The model under review builds one solid part; all positions refer to its coordinate system, in mm. Face numbers are marked on the shaded views. A direction names the side the tool comes from. Give positions to 0.01 mm unless a question says otherwise; leave off trailing zeros. Loops run counter-clockwise (first coordinate to the right, second up) from the corner with the lowest first, then second, coordinate; pieces in that order, holes last. Notation, with made-up numbers: M 70.5,61 L 105.5,61 A32 cw 105.5,88 Z; hole C 30.25,62 d3. An arc over 180 degrees is marked long. Return JSON: item names as keys, results as strings.
```python
from build123d import *

# Parameters (mm, degrees)
SKETCH_3_W          = 50
SKETCH_3_H          = 7
EXTRUDE_1_DEPTH     = 33
EXTRUDE_2_DEPTH     = 33
SKETCH_5_R          = 1.25
CUT_EXTRUDE_1_DEPTH = 8
SKETCH_6_W          = 50
SKETCH_6_H          = 4
CUT_EXTRUDE_2_DEPTH = 40
CUT_EXTRUDE_START   = -8
SKETCH_7_R          = 1.25
CUT_EXTRUDE_3_DEPTH = 8


with BuildPart() as part:
    # 草图3 → 凸台-拉伸1 (new body)
    with BuildSketch(Plane.XY):
        with Locations((25, 25)):
            Rectangle(SKETCH_3_W, SKETCH_3_H)
    extrude(amount=EXTRUDE_1_DEPTH)

    # 草图4 → 凸台-拉伸2 (add)
    with BuildSketch(Plane(origin=(0, 0, 0), x_dir=(-1, 0, 0), z_dir=(0, 0, -1))):
        with BuildLine():
            Line((-50, 21.5), (-50, 11))
            ThreePointArc((-50, 11), (-47.86188219, 17.51667431), (-42.278719262, 21.5))
            Line((-42.278719262, 21.5), (-50, 21.5))
        make_face()
        with BuildLine():
            Line((-7.721280738, 21.5), (0, 21.5))
            Line((0, 21.5), (0, 11))
            ThreePointArc((0, 11), (-2.13811781, 17.51667431), (-7.721280738, 21.5))
        make_face()
        with BuildLine():
            Line((0, 28.5), (0, 39))
            ThreePointArc((0, 39), (-2.13811781, 32.48332569), (-7.721280738, 28.5))
            Line((-7.721280738, 28.5), (0, 28.5))
        make_face()
        with BuildLine():
            Line((-50, 28.5), (-42.278719262, 28.5))
            ThreePointArc((-42.278719262, 28.5), (-47.86188219, 32.48332569), (-50, 39))
            Line((-50, 39), (-50, 28.5))
        make_face()
    extrude(amount=-EXTRUDE_2_DEPTH)

    # 草图5 → 切除-拉伸1 (cut)
    with BuildSketch(Plane(origin=(0, 0, 0), x_dir=(-1, 0, 0), z_dir=(0, 0, -1))):
        with Locations((-46.372516673, 28)):
            Circle(SKETCH_5_R)
        with Locations((-46.372516673, 22)):
            Circle(SKETCH_5_R)
        with Locations((-37.264513071, 25)):
            Circle(SKETCH_5_R)
        with Locations(Location((-3.627483327, 22, 0), (0, 0, 180))):
            Circle(SKETCH_5_R)
        with Locations(Location((-3.627483327, 28, 0), (0, 0, 180))):
            Circle(SKETCH_5_R)
        with Locations(Location((-12.735486929, 25, 0), (0, 0, 180))):
            Circle(SKETCH_5_R)
    extrude(amount=-CUT_EXTRUDE_1_DEPTH, mode=Mode.SUBTRACT)

    # 草图6 → 切除-拉伸2 (cut)
    with BuildSketch(Plane(origin=(0, 0, 0), x_dir=(-1, 0, 0), z_dir=(0, 0, -1))):
        with Locations((-25, 37)):
            Rectangle(SKETCH_6_W, SKETCH_6_H)
        with Locations((-25, 13)):
            Rectangle(SKETCH_6_W, SKETCH_6_H)
    extrude(amount=-CUT_EXTRUDE_2_DEPTH, mode=Mode.SUBTRACT)

    # 草图7 → 切除-拉伸3 (cut)
    with BuildSketch(Plane.XY.offset(33).offset(CUT_EXTRUDE_START)):
        with Locations((3.627483327, 28)):
            Circle(SKETCH_7_R)
        with Locations((3.627483327, 22)):
            Circle(SKETCH_7_R)
        with Locations((12.735486929, 25)):
            Circle(SKETCH_7_R)
        with Locations(Location((46.372516673, 22, 0), (0, 0, 180))):
            Circle(SKETCH_7_R)
        with Locations(Location((46.372516673, 28, 0), (0, 0, 180))):
            Circle(SKETCH_7_R)
        with Locations(Location((37.264513071, 25, 0), (0, 0, 180))):
            Circle(SKETCH_7_R)
    extrude(amount=CUT_EXTRUDE_3_DEPTH, mode=Mode.SUBTRACT)


solid = part.part
```
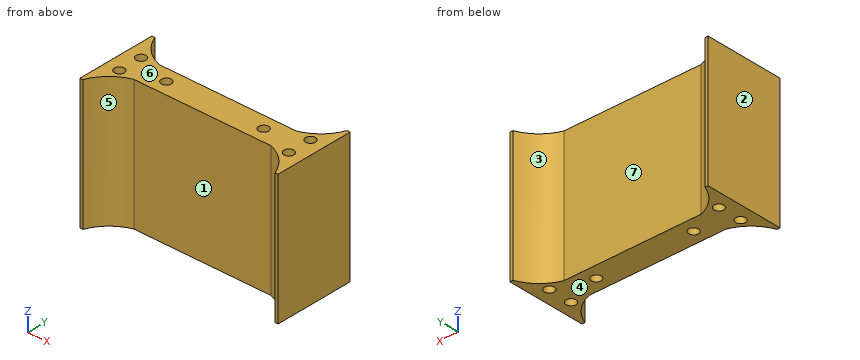
1) Insertion check: pin 1 (2 mm diameter, centred on x = 3.63, y = 28, fed in from +Z); pin 2 (1.2 mm diameter, centred on x = 12.5, y = 25, fed in from -Z); pin 3 (4 mm diameter, centred on x = 31, y = 19, fed in from -Z). Each pin has a flat end and moves straight along its axis. Give the tip position at first contact, or say it passes through.
From the geometry:
{"pin 1": "z = 25", "pin 2": "z = 8", "pin 3": "through"}
2) Consider section B-B on y = 19.5. Write out the cut boundary in (x, z), then the cut area to 3 significant figures.
From the geometry:
{"outline": "M 0,0 L 4.02,0 L 4.02,33 L 0,33 Z; M 45.98,0 L 50,0 L 50,33 L 45.98,33 Z", "area": "265 mm²"}
3) Consider section C-C on y = 25. Write out the cut boundary in (x, z), then the cut area to 3 significant figures.
From the geometry:
{"outline": "M 0,0 L 11.49,0 L 11.49,8 L 13.99,8 L 13.99,0 L 36.01,0 L 36.01,8 L 38.51,8 L 38.51,0 L 50,0 L 50,33 L 38.51,33 L 38.51,25 L 36.01,25 L 36.01,33 L 13.99,33 L 13.99,25 L 11.49,25 L 11.49,33 L 0,33 Z", "area": "1,570 mm²"}
4) Tool access review of the marked faces 5, 6 and 7: name each direction out of +Z, -Z, +X, -X, +Y, -Y from which nothing blocks a thin tool from reaching the whole face with its end or side.
From the geometry:
{"face 5": "+Z, -Z, -Y", "face 6": "+Z, +X, -X, +Y, -Y", "face 7": "+Z, -Z, +Y"}
5) Consider section D-D on z = 23. Write out the cut boundary in (x, y).
From the geometry:
{"outline": "M 0,15 L 0.75,15 A11 cw 7.72,21.5 L 42.28,21.5 A11 cw 49.25,15 L 50,15 L 50,35 L 49.25,35 A11 cw 42.28,28.5 L 7.72,28.5 A11 cw 0.75,35 L 0,35 Z"}
6) The part is to be moulded in two halves that separate along X. For the marked faces 1, 2, 3 and 4, say which applies: released by +X, released by -X, zero draft, split by the parting line, or undercut.
From the geometry:
{"face 1": "undercut", "face 2": "released by -X", "face 3": "undercut", "face 4": "zero draft"}
7) Consider section A-A on z = 27. Write out the cut boundary in (x, y).
From the geometry:
{"outline": "M 0,15 L 0.75,15 A11 cw 7.72,21.5 L 42.28,21.5 A11 cw 49.25,15 L 50,15 L 50,35 L 49.25,35 A11 cw 42.28,28.5 L 7.72,28.5 A11 cw 0.75,35 L 0,35 Z; hole C 3.63,22 d2.5; hole C 3.63,28 d2.5; hole C 12.74,25 d2.5; hole C 37.26,25 d2.5; hole C 46.37,22 d2.5; hole C 46.37,28 d2.5"}
8) Wall thickness on L1, parallel to Y at x = 34, z = 10.5; L2, parallel to X at y = 33.75, z = 11.5; L3, parallel to Y at x = 4.5, z = 29: over which ranges is each line inside the solid? List them lowest first. Write a range as from..to.
From the geometry:
{"L1": "21.5..28.5", "L2": "0..1.33, 48.67..50", "L3": "19.87..21.1, 22.9..27.1, 28.9..30.13"}
